```python
from build123d import *

# Parameters (mm, degrees)
SKETCH_1_R          = 5
EXTRUDE_1_DEPTH     = 52
SKETCH_2_R          = 3.5
EXTRUDE_2_DEPTH     = 2
SKETCH_3_R          = 5
EXTRUDE_3_DEPTH     = 14
SKETCH_4_R          = 5
EXTRUDE_4_DEPTH     = 2
SKETCH_5_R          = 5
EXTRUDE_5_DEPTH     = 4
SKETCH_6_R          = 5
EXTRUDE_6_DEPTH     = 2
SKETCH_7_R          = 5
EXTRUDE_7_DEPTH     = 10
EXTRUDE_START       = 2
SKETCH_8_R          = 3.5
EXTRUDE_8_DEPTH     = 2
EXTRUDE_START_2     = 14
SKETCH_9_R          = 5
EXTRUDE_9_DEPTH     = 14
SKETCH_10_R         = 5
EXTRUDE_10_DEPTH    = 2
EXTRUDE_START_3     = 4
SKETCH_11_R         = 5
EXTRUDE_11_DEPTH    = 4
SKETCH_12_R         = 5
EXTRUDE_12_DEPTH    = 2
EXTRUDE_START_4     = 10
SKETCH_13_R         = 5
EXTRUDE_13_DEPTH    = 10
CHAMFER_1_SIZE      = 0.5
CUT_EXTRUDE_START   = -2
SKETCH_14_R         = 5
SKETCH_14_R_2       = 3.5
CUT_EXTRUDE_1_DEPTH = 2
SKETCH_15_R         = 5
SKETCH_15_R_2       = 3.5
CUT_EXTRUDE_2_DEPTH = 2
CUT_EXTRUDE_START_2 = -15
SKETCH_16_R         = 5
CUT_EXTRUDE_3_DEPTH = 15
SKETCH_17_R         = 5
CUT_EXTRUDE_4_DEPTH = 15
CHAMFER_2_SIZE      = 0.5


with BuildPart() as part:
    # 草图1 → 凸台-拉伸1 (new body)
    with BuildSketch(Plane(origin=(0, 0, 0), x_dir=(0, 0, -1), z_dir=(1, 0, 0))):
        with Locations(Location((0, 0, 0), (0, 0, 180))):
            Circle(SKETCH_1_R)
    extrude(amount=EXTRUDE_1_DEPTH)

    # 草图2 → 凸台-拉伸2 (add)
    with BuildSketch(Plane(origin=(52, 0, 0), x_dir=(0, 0, -1), z_dir=(1, 0, 0))):
        Circle(SKETCH_2_R)
    extrude(amount=EXTRUDE_2_DEPTH)

    # 草图3 → 凸台-拉伸3 (add)
    with BuildSketch(Plane(origin=(54, 0, 0), x_dir=(0, 0, -1), z_dir=(1, 0, 0))):
        with Locations(Location((0, 0, 0), (0, 0, 180))):
            Circle(SKETCH_3_R)
    extrude(amount=EXTRUDE_3_DEPTH)

    # 草图4 → 凸台-拉伸4 (add)
    with BuildSketch(Plane(origin=(68, 0, 0), x_dir=(0, 0, -1), z_dir=(1, 0, 0))):
        with Locations(Location((0, 0, 0), (0, 0, 180))):
            Circle(SKETCH_4_R)
    extrude(amount=EXTRUDE_4_DEPTH)

    # 草图5 → 凸台-拉伸5 (add)
    with BuildSketch(Plane(origin=(70, 0, 0), x_dir=(0, 0, -1), z_dir=(1, 0, 0))):
        with Locations(Location((0, 0, 0), (0, 0, 180))):
            Circle(SKETCH_5_R)
    extrude(amount=EXTRUDE_5_DEPTH)

    # 草图6 → 凸台-拉伸6 (add)
    with BuildSketch(Plane(origin=(74, 0, 0), x_dir=(0, 0, -1), z_dir=(1, 0, 0))):
        with Locations(Location((0, 0, 0), (0, 0, 180))):
            Circle(SKETCH_6_R)
    extrude(amount=EXTRUDE_6_DEPTH)

    # 草图7 → 凸台-拉伸7 (add)
    with BuildSketch(Plane(origin=(76, 0, 0), x_dir=(0, 0, -1), z_dir=(1, 0, 0))):
        with Locations(Location((0, 0, 0), (0, 0, 180))):
            Circle(SKETCH_7_R)
    extrude(amount=EXTRUDE_7_DEPTH)

    # 草图8 → 凸台-拉伸8 (add)
    with BuildSketch(Plane.ZY.offset(EXTRUDE_START)):
        with Locations(Location((0, 0, 0), (0, 0, 180))):
            Circle(SKETCH_8_R)
    extrude(amount=-EXTRUDE_8_DEPTH)

    # 草图9 → 凸台-拉伸9 (add)
    with BuildSketch(Plane.ZY.offset(2).offset(EXTRUDE_START_2)):
        Circle(SKETCH_9_R)
    extrude(amount=-EXTRUDE_9_DEPTH)

    # 草图10 → 凸台-拉伸10 (add)
    with BuildSketch(Plane.ZY.offset(16).offset(EXTRUDE_START)):
        Circle(SKETCH_10_R)
    extrude(amount=-EXTRUDE_10_DEPTH)

    # 草图11 → 凸台-拉伸11 (add)
    with BuildSketch(Plane.ZY.offset(18).offset(EXTRUDE_START_3)):
        Circle(SKETCH_11_R)
    extrude(amount=-EXTRUDE_11_DEPTH)

    # 草图12 → 凸台-拉伸12 (add)
    with BuildSketch(Plane.ZY.offset(22).offset(EXTRUDE_START)):
        Circle(SKETCH_12_R)
    extrude(amount=-EXTRUDE_12_DEPTH)

    # 草图13 → 凸台-拉伸13 (add)
    with BuildSketch(Plane.ZY.offset(24).offset(EXTRUDE_START_4)):
        Circle(SKETCH_13_R)
    extrude(amount=-EXTRUDE_13_DEPTH)

    # 倒角1
    chamfer_1_edges = [part.edges().sort_by_distance(p)[0] for p in [
        (86, 0, -5),
        (-34, 0, -5),
    ]]
    chamfer(chamfer_1_edges, length=CHAMFER_1_SIZE)

    # 草图14 → 切除-拉伸1 (cut)
    with BuildSketch(Plane(origin=(-8, 0, 0), x_dir=(0, 0, -1), z_dir=(1, 0, 0)).offset(CUT_EXTRUDE_START)):
        with Locations(Location((0, 0, 0), (0, 0, 180))):
            Circle(SKETCH_14_R)
        Circle(SKETCH_14_R_2, mode=Mode.SUBTRACT)
    cut_extrude_1 = extrude(amount=CUT_EXTRUDE_1_DEPTH, mode=Mode.SUBTRACT)

    # 草图15 → 切除-拉伸2 (cut)
    with BuildSketch(Plane(origin=(-14, 0, 0), x_dir=(0, 0, -1), z_dir=(1, 0, 0)).offset(CUT_EXTRUDE_START)):
        with Locations(Location((0, 0, 0), (0, 0, 180))):
            Circle(SKETCH_15_R)
        Circle(SKETCH_15_R_2, mode=Mode.SUBTRACT)
    cut_extrude_2 = extrude(amount=CUT_EXTRUDE_2_DEPTH, mode=Mode.SUBTRACT)

    # 镜向1: 切除-拉伸1, 切除-拉伸2 across plane
    add(cut_extrude_1.mirror(Plane(origin=(26, 0, 0), x_dir=(0, 0, 1), z_dir=(1, 0, 0))), mode=Mode.SUBTRACT)
    add(cut_extrude_2.mirror(Plane(origin=(26, 0, 0), x_dir=(0, 0, 1), z_dir=(1, 0, 0))), mode=Mode.SUBTRACT)

    # 草图16 → 切除-拉伸3 (cut)
    with BuildSketch(Plane(origin=(86, 0, 0), x_dir=(0, 0, -1), z_dir=(1, 0, 0)).offset(CUT_EXTRUDE_START_2)):
        Circle(SKETCH_16_R)
    extrude(amount=CUT_EXTRUDE_3_DEPTH, mode=Mode.SUBTRACT)

    # 草图17 → 切除-拉伸4 (cut)
    with BuildSketch(Plane.ZY.offset(34)):
        with Locations(Location((0, 0, 0), (0, 0, 180))):
            Circle(SKETCH_17_R)
    extrude(amount=-CUT_EXTRUDE_4_DEPTH, mode=Mode.SUBTRACT)

    # 倒角2
    chamfer_2_edges = [part.edges().sort_by_distance(p)[0] for p in [
        (-19, 0, -5),
        (71, 0, -5),
    ]]
    chamfer(chamfer_2_edges, length=CHAMFER_2_SIZE)


solid = part.part
```
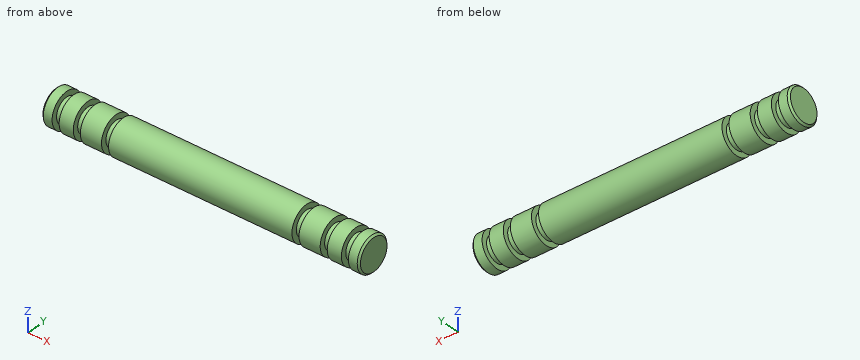
Model file for the job. Use its own axes, mm. Give positions to 0.01 mm unless a question says otherwise; leave off trailing zeros. Order: outer loops, then holes, each group sorted by start corner. A loop starts at its lowest first (then second) coordinate and runs counter-clockwise, first axis right, second up.
1) Wall check: probe 1 along Z at (x, y) = (61, -1); probe 2 along Y at (x, z) = (51.5, 4.5); probe 3 along Z at (x, y) = (-12, -1.75). Give the ranges that are in metal, low to high.
2) Pin check, flat tips, straight feed: pin 1 (1 mm diameter, centred on x = 6.5, z = -3.5, fed in from -Y); pin 2 (3 mm diameter, centred on x = 28.5, z = -3, fed in from -Y); pin 3 (4 mm diameter, centred on x = 5.5, z = 2.5, fed in from -Y). Stop position of each tip, or through.
3) Saw through at A-A, the plane x = -12.5. Write the cut outline in (y, z).
Computed:
1. probe 1: z = -3.35 to 3.35
1. probe 2: y = -2.18 to 2.18
1. probe 3: z = -4.68 to 4.68
2. pin 1: stops at y = -4
2. pin 2: stops at y = -4.77
2. pin 3: stops at y = -4.97
3. outline: circle Ø10 at (0, 0)
